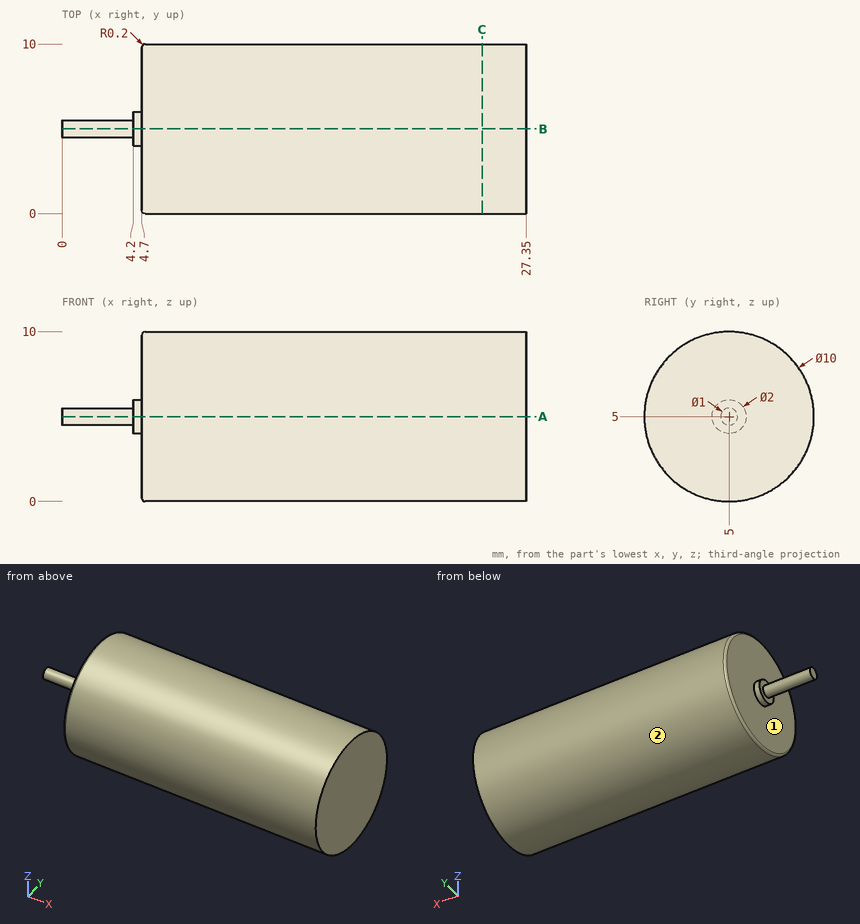
The drawing under review shows one solid part. Ordinate dimensions are in mm from its lowest x, y, z. A direction names the side the tool comes from. Round coordinates to 2 decimals unless told otherwise and drop trailing zeros. Loops run counter-clockwise (first coordinate to the right, second up) from the corner with the lowest first, then second, coordinate; pieces in that order, holes last. Notation, with made-up numbers: (-13, -26) - (0, -26) arc R12 cw to (0, -17) - close; hole circle Ø6 at (55, 52.5). An arc over 180 degrees is marked (long way). One line per item, written item: value. Start each with the question number.
1) Insertion check: pin 1 Ø3 at (x, y) = (12, 3) entering from +Z; pin 2 Ø2 at (y, z) = (6.5, 6.5) entering from -X; pin 3 Ø1.5 at (x, z) = (16.5, 8.5) entering from -Y. Each pin has a flat end and moves straight along its axis. Give the tip position at first contact, or say it passes through.
2) For the marked faces 1 and 2, list the 3-axis set-ups (+Z, -Z, +X, -X, +Y, -Y) from which the entire face can be reached by the end or side of a thin tool; tool diameter is ignored.
3) To check wall thickness, follow L1, parallel to X at y = 5, z = 3; L2, parallel to Z at x = 8.5, y = 5.25; L3, parallel to X at y = 5.25, z = 5.5. State the ranges of each line that lie inside material, in increasing order. Write a range as from..to.
4) Consider section A-A on z = 5. Give the boundary of the cut face in (x, y), then the cut area to 3 significant figures.
5) Consider section C-C on x = 24.75. Give the boundary of the cut face in (y, z).
Reported:
1. pin 1: stops at z = 9.97
1. pin 2: stops at x = 4.7
1. pin 3: stops at y = 0.82
2. face 1: -X
2. face 2: +X, -X
3. L1: x = 4.7..27.35
3. L2: z = 0.01..9.99
3. L3: x = 4.2..27.35
4. outline: (0, 4.5) - (4.2, 4.5) - (4.2, 4) - (4.7, 4) - (4.7, 0.2) arc R0.2 ccw to (4.9, 0) - (27.35, 0) - (27.35, 10) - (4.9, 10) arc R0.2 ccw to (4.7, 9.8) - (4.7, 6) - (4.2, 6) - (4.2, 5.5) - (0, 5.5) - close
4. area: 232 mm^2
5. outline: circle Ø10 at (5, 5)
